Autodesk Inventor part; units mm, degrees
ref_plane "bolt_XY" through (5, 0, 0) normal (1, 0, 0) x (0, 0, -1)
ref_plane "bolt_YZ" through (5, 0, 0) normal (0, 0, -1) x (0, 1, 0)
ref_plane "bolt_ZX" through (5, 0, 0) normal (0, 1, 0) x (1, 0, 0)
sketch "Sketch_1" plane through (0, 0, 0) normal (0, 0, 1) x (1, 0, 0)
  line L0 (5, 0) -> (-3, 0)
  line L1 (-3, 0) -> (-3, 2.45)
  line L2 (-3, 2.45) -> (-2.7, 2.75)
  line L3 (-2.7, 2.75) -> (0, 2.75)
  line L4 (0, 2.75) -> (0, 1.5)
  line L5 (0, 1.5) -> (4.6935, 1.5)
  line L6 (4.6935, 1.5) -> (5, 1.1935)
  line L7 (5, 1.1935) -> (5, 0)
  line L8 (5, 0) -> (-3, 0)
revolve "Revolution1" add sketch "Sketch_1" angle 360 about axis through (5, 0, 0) along (1, 0, 0)
thread "Thread1"
sketch "Sketch2" plane through (-3, 0, 0) normal (-1, 0, 0) x (0, 0, 1)
  point P0 (0, 0)
hole "Hole1" at (-3, 0, 0) direction (1, 0, 0) diameter 2.5 depth 1.3 tip angle 120
sketch "Sketch_3" plane through (-3, 0, 0) normal (1, 0, 0) x (0, 0, -1)
  line L0 (-1.25, -0.7217) -> (0, -1.4434)
  line L1 (0, -1.4434) -> (1.25, -0.7217)
  line L2 (1.25, -0.7217) -> (1.25, 0.7217)
  line L3 (1.25, 0.7217) -> (0, 1.4434)
  line L4 (0, 1.4434) -> (-1.25, 0.7217)
  line L5 (-1.25, 0.7217) -> (-1.25, -0.7217)
extrude "Extrusion1" cut sketch "Sketch_3" along normal blind 1.3
ref_plane "bolt_XY" through (5, 0, 0) normal (1, 0, 0) x (0, 0, -1)
ref_plane "bolt_YZ" through (5, 0, 0) normal (0, 0, -1) x (0, 1, 0)
ref_plane "bolt_ZX" through (5, 0, 0) normal (0, 1, 0) x (1, 0, 0)
ref_plane "nut_XY" through (0, 0, 0) normal (1, 0, 0) x (0, 0, -1)
ref_plane "nut_YZ" through (0, 0, 0) normal (0, 0, -1) x (0, 1, 0)
ref_plane "nut_ZX" through (0, 0, 0) normal (0, 1, 0) x (1, 0, 0)
properties part number "CBE3-5"
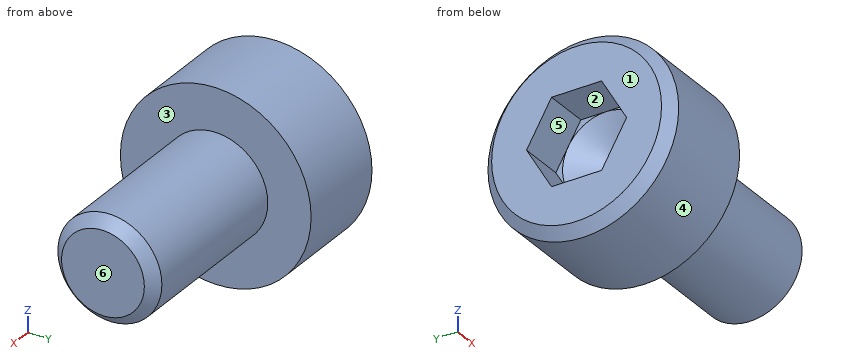
Could you check a few things on this model? Use its own coordinates, in mm. Face numbers are marked on the shaded views. A direction names the side the tool comes from. Round coordinates to 2 decimals unless told otherwise and drop trailing zeros. Order: outer loops, then holes, each group sorted by start corner. A loop starts at its lowest first (then second) coordinate and runs counter-clockwise, first axis right, second up. Notation, with made-up numbers: M 6.25,21 L 32.25,21 A16 ccw 32.25,45 Z; hole C -12,47 d8. An arc over 180 degrees is marked long. One line per item, written item: value.
(1) If we mould it in two halves opening along Z, with no side actions, what happens to the marked faces 4, 5 and 6? For each: released by +Z, released by -Z, zero draft, split by the parting line, or undercut.
Ans:
face 4: split by the parting line
face 5: undercut
face 6: zero draft
(2) Imagine slicing it at A-A (x = -1.25). Write out the boundary of the cut face in (y, z).
Ans:
outline: C 0,0 d5.5; hole C 0,0 d0.94
(3) Imagine slicing it at B-B (x = -0.25). Write out the boundary of the cut face in (y, z), and give its area (3 significant figures).
Ans:
outline: C 0,0 d5.5
area: 23.8 mm^2
(4) Which directions (+Z, -Z, +X, -X, +Y, -Y) give clear straight access to the entire face, cutting with the end or side of a thin tool? Please do the marked faces 1, 2 and 3.
Ans:
face 1: +Z, -Z, -X, +Y, -Y
face 2: -X
face 3: +X
(5) I need wall thicknesses on line 1 along X through (y, z) = (2.1, 0.8); line 2 along Y through (x, z) = (-0.25, 0.1); line 3 along Z through (x, y) = (0.5, -0.5). Which ranges of each line are inside material? Lowest first, please. Write a range as from..to.
Ans:
line 1: x = -3..0
line 2: y = -2.75..2.75
line 3: z = -1.41..1.41
(6) Imagine slicing it at C-C (x = 3). Write out the boundary of the cut face in (y, z).
Ans:
outline: C 0,0 d3
